from build123d import *

# Parameters (mm, degrees)
SKETCH1_R           = 6.25
BOSS_EXTRUDE1_DEPTH = 20
SKETCH2_R           = 8
BOSS_EXTRUDE2_DEPTH = 8
SKETCH3_W           = 16
SKETCH3_H           = 332.488311808
CUT_EXTRUDE1_DEPTH  = 90


with BuildPart() as part:
    # Sketch1 → Boss-Extrude1 (new, symmetric)
    with BuildSketch(Plane.XY):
        with BuildLine():
            Line((0, -25), (85, -25))
            ThreePointArc((85, -25), (109.985084644, 0.943739672), (83.11944661, 24.934770827))
            ThreePointArc((83.11944661, 24.934770827), (44.228399081, 29.699192353), (10.153265793, 49.040820564))
            Line((10.153265793, 49.040820564), (-33.31339639, 37.393963534))
            Line((-33.31339639, 37.393963534), (-20.890082225, -8.970476128))
            ThreePointArc((-20.890082225, -8.970476128), (-13.165686186, -20.530851753), (0, -25))
        make_face()
        Circle(SKETCH1_R, mode=Mode.SUBTRACT)
        with BuildLine():
            Line((85.000943792, -13.497203546), (45.00094389, -13.499999967))
            ThreePointArc((45.00094389, -13.499999967), (31.500000131, -0.000943792), (44.999056306, 13.499999967))
            Line((44.999056306, 13.499999967), (84.999056208, 13.502796388))
            ThreePointArc((84.999056208, 13.502796388), (98.499999967, 0.003740213), (85.000943792, -13.497203546))
        make_face(mode=Mode.SUBTRACT)
    extrude(amount=BOSS_EXTRUDE1_DEPTH, both=True)

    # Sketch2 → Boss-Extrude2 (add, symmetric)
    with BuildSketch(Plane.XY):
        with BuildLine():
            Line((-33.31339639, 37.393963534), (-42.372062969, 71.201367454))
            ThreePointArc((-42.372062969, 71.201367454), (-28.229927345, 95.696264882), (-3.735029917, 81.554129259))
            Line((-3.735029917, 81.554129259), (5.323636662, 47.746725338))
            Line((5.323636662, 47.746725338), (-33.31339639, 37.393963534))
        make_face()
        with Locations((-23.053546443, 76.377748356)):
            Circle(SKETCH2_R, mode=Mode.SUBTRACT)
    extrude(amount=BOSS_EXTRUDE2_DEPTH, both=True)

    # Sketch3 → Cut-Extrude1 (cut)
    with BuildSketch(Plane(origin=(109.985084644, 0, 0), x_dir=(0, 0, -1), z_dir=(1, 0, 0))):
        with Locations((0, -25)):
            Rectangle(SKETCH3_W, SKETCH3_H)
    extrude(amount=-CUT_EXTRUDE1_DEPTH, mode=Mode.SUBTRACT)


solid = part.part
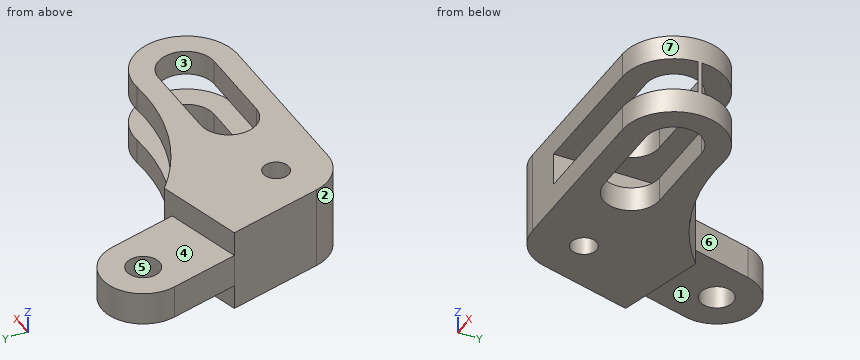
Design review of the part built by this model. Coordinates are the model's own, in mm. Face numbers are marked on the shaded views. A direction names the side the tool comes from. Round coordinates to 2 decimals unless told otherwise and drop trailing zeros. Write each loop counter-clockwise with the first axis right and the second up, starting at its lowest first coordinate (ties: lowest second). Pieces come first, ordered by that corner, then holes. Notation, with made-up numbers: (-39.75, 16) -> (15.25, 16) arc R13 cw to (15.25, 23) -> close; hole circle Ø6 at (15.25, 74). An arc over 180 degrees is marked (long way). One line per item, written item: value. Start each with the question number.
Q1. Add section B-B (z = -2). Give the boundary of the cut face in (x, y), then the cut area to 3 significant figures.
Q2. Add section C-C (z = -12.5). Give the boundary of the cut face in (x, y), then the cut area to 3 significant figures.
Q3. Add section D-D (y = 22.5). Give the boundary of the cut face in (x, z), then the cut area to 3 significant figures.
Q4. The part is to be moulded in two halves that separate along Y. For the marked faces 4, 5, 6 and 7, say which applies: pulls with the +Y half, pulls with the -Y half, needs draft (parallel to the pull), parting line crosses it, or undercut.
Q5. To check wall thickness, follow probe 1 along Z at (x, y) = (50.5, -19); probe 2 along Y at (x, z) = (75, -11.5); probe 3 along X at (y, z) = (10, -17.5). State the ranges of each line that lie inside material, in increasing order.
Q6. Insertion check: P1, Ø13, axis at x = 58.5, z = -14.5, coming from the +Y side; P2, Ø0.9, axis at y = 0, z = 2, coming from the -X side; P3, Ø24, axis at x = -27.5, y = 52.5, coming from the -Z side. Each pin has a flat end and moves straight along its axis. Give the tip position at first contact, or say it passes through.
Q7. Tool access review of the marked faces 1, 2 and 3: name each direction out of +Z, -Z, +X, -X, +Y, -Y from which nothing blocks a thin tool from reaching the whole face with its end or side.
Q8. Add section A-A (x = 37). Give the boundary of the cut face in (y, z).
Response:
1. outline: (-42.37, 71.2) -> (-20.89, -8.97) arc R21.63 ccw to (0, -25) -> (19.99, -25) -> (19.99, 41.54) arc R100 cw to (10.15, 49.04) -> (5.32, 47.75) -> (-3.74, 81.55) arc R20 ccw to start; (109.99, -0.94) arc R25 ccw to (109.99, 0.94) -> close; hole circle Ø16 at (-23.05, 76.38); hole circle Ø12.5 at (0, 0)
1. area: 4,780 mm^2
2. outline: (-33.31, 37.39) -> (-20.89, -8.97) arc R21.63 ccw to (0, -25) -> (85, -25) arc R25 ccw (long way) to (83.12, 24.93) arc R100 cw to (10.15, 49.04) -> close; hole circle Ø12.5 at (0, 0); hole (45, -13.5) -> (85, -13.5) arc R13.5 ccw to (85, 13.5) -> (45, 13.5) arc R13.5 ccw to start
2. area: 5,820 mm^2
3. outline: (-29.32, -20) -> (95.91, -20) -> (95.91, -8) -> (19.99, -8) -> (19.99, 8) -> (95.91, 8) -> (95.91, 20) -> (-29.32, 20) -> close
3. area: 3,790 mm^2
4. face 4: needs draft
4. face 5: undercut
4. face 6: pulls with the +Y half
4. face 7: parting line crosses it
5. probe 1: z = -20 to -8, 8 to 20
5. probe 2: y = -25 to -13.5, 13.5 to 24.65
5. probe 3: x = -25.97 to 35.93, 94.07 to 107.92
6. P1: stops at y = 27.48
6. P2: stops at x = -23.41
6. P3: stops at z = -8
7. face 1: -Z, -X, +Y
7. face 2: +Z, -Z, -X, -Y
7. face 3: +Z, -Z
8. outline: (-25, -20) -> (-10.87, -20) -> (-10.87, -8) -> (-25, -8) -> close; (-25, 8) -> (-10.87, 8) -> (-10.87, 20) -> (-25, 20) -> close; (10.87, -20) -> (32.4, -20) -> (32.4, -8) -> (10.87, -8) -> close; (10.87, 8) -> (32.4, 8) -> (32.4, 20) -> (10.87, 20) -> close
